For this review, use the dimensioned drawing (mm, ordinates from the lowest corner) and the shaded views. A direction names the side the tool comes from. Round coordinates to 2 decimals unless told otherwise and drop trailing zeros. Write each loop counter-clockwise with the first axis right and the second up, starting at its lowest first coordinate (ties: lowest second). Pieces come first, ordered by that corner, then holes.
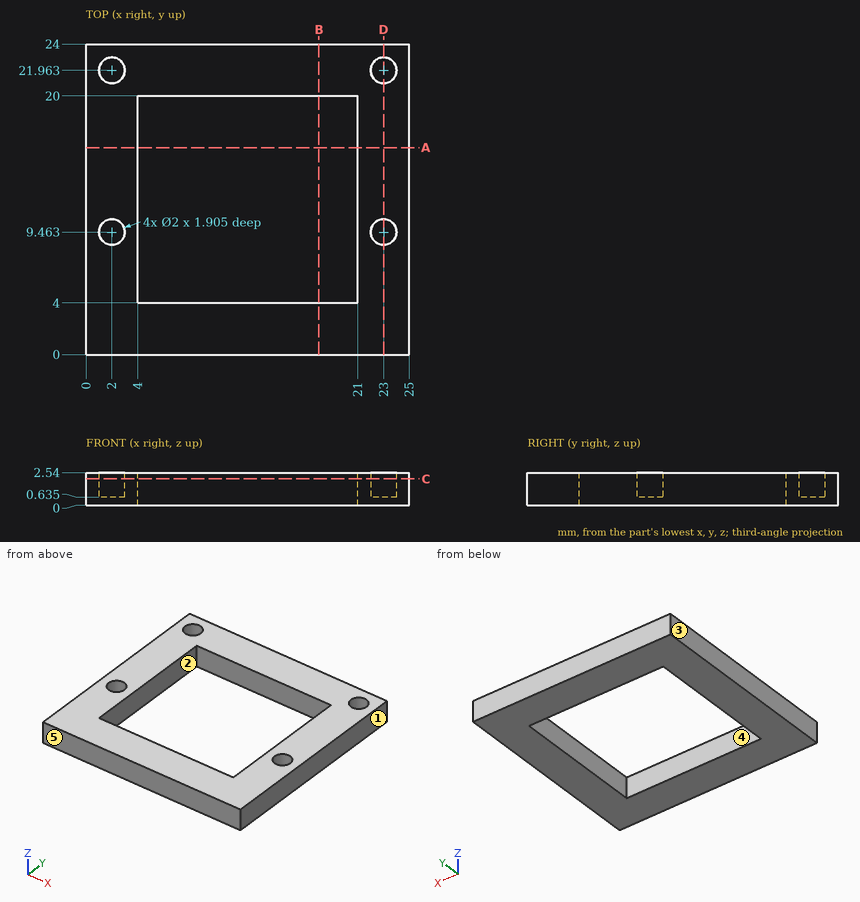
(1) We need section A-A, the plane y = 16. Give the boundary of the cut face in (x, z).
Geometry check:
outline: (0, 0) - (4, 0) - (4, 2.54) - (0, 2.54) - close; (21, 0) - (25, 0) - (25, 2.54) - (21, 2.54) - close
(2) For line 1 along Y through (x, z) = (2, 1.7); line 2 along Y through (x, z) = (17, 2.05); line 3 along X through (y, z) = (16, 1), list the stretches that pass through material, from the lowest coordinate up.
Geometry check:
line 1: y = 0 to 8.46, 10.46 to 20.96, 22.96 to 24
line 2: y = 0 to 4, 20 to 24
line 3: x = 0 to 4, 21 to 25
(3) We need section D-D, the plane x = 23. Give the boundary of the cut face in (y, z) (1 decimal).
Geometry check:
outline: (0, 0) - (24, 0) - (24, 2.5) - (23, 2.5) - (23, 0.6) - (21, 0.6) - (21, 2.5) - (10.5, 2.5) - (10.5, 0.6) - (8.5, 0.6) - (8.5, 2.5) - (0, 2.5) - close
(4) Mouldability with a two-part tool opening along X and no side actions: class the marked faces 3, 4 and 5 as pulls with the +X half, pulls with the -X half, needs draft (parallel to the pull), parting line crosses it, or undercut.
Geometry check:
face 3: pulls with the -X half
face 4: undercut
face 5: needs draft
(5) We need section B-B, the plane x = 18. Give the boundary of the cut face in (y, z), and give its area (3 significant figures).
Geometry check:
outline: (0, 0) - (4, 0) - (4, 2.54) - (0, 2.54) - close; (20, 0) - (24, 0) - (24, 2.54) - (20, 2.54) - close
area: 20.3 mm2
(6) We need section C-C, the plane z = 2.05. Give the boundary of the cut face in (x, y).
Geometry check:
outline: (0, 0) - (25, 0) - (25, 24) - (0, 24) - close; hole circle Ø2 at (2, 9.46); hole circle Ø2 at (2, 21.96); hole (4, 4) - (21, 4) - (21, 20) - (4, 20) - close; hole circle Ø2 at (23, 9.46); hole circle Ø2 at (23, 21.96)
(7) For the marked faces 1 and 2, list the 3-axis set-ups (+Z, -Z, +X, -X, +Y, -Y) from which the entire face can be reached by the end or side of a thin tool; tool diameter is ignored.
Geometry check:
face 1: +Z, -Z, +X, +Y, -Y
face 2: +Z, -Z
(8) For pin 1 Ø0.6 at (x, y) = (23.5, 9.5) entering from +Z (3 decimals), flat-tipped, find the tip position at first contact; note if it passes through.
Geometry check:
pin 1: stops at z = 0.635
